from build123d import *

# Parameters (mm, degrees)
F1_DEPTH = 15.875
F3_DEPTH = 25.4
F5_DEPTH = 25.4


with BuildPart() as f1:
    # F0 (on Top) → F1 (new body)
    with BuildSketch(Plane.XY):
        Polygon((0, 466.725), (488.95, -22.225), (854.075, -22.225), (854.075, 831.85), (0, 831.85), align=None)
    extrude(amount=-F1_DEPTH)

    # F2 (on face) → F3 (cut)
    with BuildSketch(Plane.XY):
        Polygon((-101.9354011834, 568.6604011834), (244.475, 222.25), (590.8854011834, -124.1604011834), (602.1107213347, -112.935081032), (257.2878201513, 231.8878201513), (254.1128201513, 235.0628201513), (-90.710081032, 579.8857213347), align=None)
    extrude(amount=-F3_DEPTH, mode=Mode.SUBTRACT)

    # F4 (on face) → F5 (cut)
    with BuildSketch(Plane.XY):
        Polygon((107.249497258, 494.179344558), (51.1228965013, 438.0527438014), (64.5932806829, 424.5823596198), (120.7198814396, 480.7089603764), align=None)
    extrude(amount=-F5_DEPTH, mode=Mode.SUBTRACT)


solid = f1.part
Geometry: final body of the model. Coordinates: model frame, mm. A direction names the side the tool comes from. Round coordinates to 2 decimals unless told otherwise and drop trailing zeros. Loops run counter-clockwise (first coordinate to the right, second up) from the corner with the lowest first, then second, coordinate; pieces in that order, holes last. Notation, with made-up numbers: (3, 2.5) -> (49, 2.5) arc R5 cw to (49, 10.5) -> close; hole circle Ø10 at (-38.5, -23). An arc over 180 degrees is marked (long way). One line per question, with ' | ' between items. Start each with the question number.
1. Mould query, pull axis X, two halves, no side actions, for faces 3 (the face through (516, 506, -15.875)), 4 (the face through (79.58, 466.51, -7.83)), 5 (the face through (25.919, 463.256, -7.826)). Classes: pulls with the +X half, pulls with the -X half, needs draft (parallel to the pull), parting line crosses it, or undercut.
2. Line query: line 1 along X through (y, z) = (288.5, -5.5) (3 decimals); line 2 along X through (y, z) = (447.5, -5.5) (3 decimals); line 3 along Y through (x, z) = (399, -1.5). Output: solid intervals per line, ascending. Write a range as [from, to].
3. Section C-C on x = 156. Output: boundary loops of the cut face in (y, z) (3 decimals).
4. Section B-B on y = 168.5. Output: boundary loops of the cut face in (x, z) (3 decimals), and give its area (3 significant figures).
5. Set-up query: faces 1 (the face through (291.125, 198.051, -7.826)), 2 (the face through (92.26, 452.25, -7.83)). Return all of +Z, -Z, +X, -X, +Y, -Y with unobstructed straight access to the full face (end or side cutting, diameter ignored); none if empty.
Returned:
1) face 3: needs draft | face 4: undercut | face 5: pulls with the -X half
2) line 1: x = [200.676, 854.075] | line 2: x = [41.676, 60.57], [87.511, 854.075] | line 3: y = [90.18, 831.85]
3) outline: (333.176, -15.875) -> (831.85, -15.875) -> (831.85, 0) -> (333.176, 0) -> close
4) outline: (320.676, -15.875) -> (854.075, -15.875) -> (854.075, 0) -> (320.676, 0) -> close | area: 8,470 mm2
5) face 1: +Z, -Z, -X, -Y | face 2: +Z, -Z
